Design review of the part built by this model. Coordinates are the model's own, in mm. Face numbers are marked on the shaded views. A direction names the side the tool comes from. Give positions to 0.01 mm unless a question says otherwise; leave off trailing zeros. Order: outer loops, then holes, each group sorted by start corner. A loop starts at its lowest first (then second) coordinate and runs counter-clockwise, first axis right, second up. Notation, with made-up numbers: (46.25, -20.75) -> (100.25, -20.75) arc R34 cw to (100.25, 13.25) -> close; hole circle Ø10 at (55.25, 16.25). An arc over 180 degrees is marked (long way). Use a Markdown table: item, result. Add a question column.
```python
from build123d import *

# Parameters (mm, degrees)
SKETCH1_W                = 177.8
SKETCH1_H                = 127
BOSS_EXTRUDE1_DEPTH      = 3.175
CONVERT_SOLID2_START     = -88.9
CONVERT_SOLID2_OUTLINE_W = 1.5875
CONVERT_SOLID2_OUTLINE_H = 127
CONVERT_SOLID2_DEPTH     = 177.8
EDGE_FLANGE1_DEPTH       = 177.8
EDGE_FLANGE2_DEPTH       = 177.8
SKETCH17_R               = 2.54
CUT_EXTRUDE1_DEPTH       = 5.08
FILLET1_R                = 12.7
SKETCH18_R               = 3.175
CUT_EXTRUDE2_DEPTH       = 5.08
SKETCH19_R               = 12.7
CUT_EXTRUDE3_DEPTH       = 12.7
SKETCH26_R               = 9.525
CUT_EXTRUDE9_DEPTH       = 5.08
SKETCH27_R               = 2.54
CUT_EXTRUDE10_DEPTH      = 5.08
SKETCH28_R               = 2.54
CUT_EXTRUDE11_DEPTH      = 5.08


# Read off the part's stored shape, not the designer's step: Convert-Solid2
# Sheet-metal steps are written as plain solids
with BuildPart() as part:
    # Sketch1 → Boss-Extrude1 (new body)
    with BuildSketch(Plane(origin=(0, 0, 0), x_dir=(1, 0, 0), z_dir=(0, 1, 0))):
        Rectangle(SKETCH1_W, SKETCH1_H)
    extrude(amount=BOSS_EXTRUDE1_DEPTH)

    # Convert-Solid2 outline → Convert-Solid2 (add)
    with BuildSketch(Plane.YZ.offset(CONVERT_SOLID2_START)):
        with Locations((-0.79375, 0)):
            Rectangle(CONVERT_SOLID2_OUTLINE_W, CONVERT_SOLID2_OUTLINE_H)
    extrude(amount=CONVERT_SOLID2_DEPTH)

    # Edge-Flange1 section (across the edge) → Edge-Flange1 (add)
    with BuildSketch(Plane(origin=(88.9, 3.175, -68.2625), x_dir=(0, 0, 1), z_dir=(-1, 0, 0))):
        with BuildLine():
            Line((-4.7625, 4.7625), (-4.7625, 33.3375))
            Line((-4.7625, 33.3375), (0, 33.3375))
            Line((0, 33.3375), (0, 4.7625))
            ThreePointArc((0, 4.7625), (1.394903955, 1.394903955), (4.7625, 0))
            Line((4.7625, 0), (4.7625, -4.7625))
            ThreePointArc((4.7625, -4.7625), (-1.972692091, -1.972692091), (-4.7625, 4.7625))
        make_face()
    extrude(amount=EDGE_FLANGE1_DEPTH)

    # Edge-Flange2 section (across the edge) → Edge-Flange2 (add)
    with BuildSketch(Plane(origin=(-88.9, 3.175, 68.2625), x_dir=(0, 0, -1), z_dir=(1, 0, 0))):
        with BuildLine():
            Line((-4.7625, 4.7625), (-4.7625, 33.3375))
            Line((-4.7625, 33.3375), (0, 33.3375))
            Line((0, 33.3375), (0, 4.7625))
            ThreePointArc((0, 4.7625), (1.394903955, 1.394903955), (4.7625, 0))
            Line((4.7625, 0), (4.7625, -4.7625))
            ThreePointArc((4.7625, -4.7625), (-1.972692091, -1.972692091), (-4.7625, 4.7625))
        make_face()
    extrude(amount=EDGE_FLANGE2_DEPTH)

    # Sketch17 → Cut-Extrude1 (cut)
    with BuildSketch(Plane(origin=(0, 0, -73.025), x_dir=(-1, 0, 0), z_dir=(0, 0, -1))):
        with Locations(Location((-76.2, 23.8125, 0), (0, 0, 90))):
            Circle(SKETCH17_R)
        with Locations(Location((-54.428571429, 23.8125, 0), (0, 0, 90))):
            Circle(SKETCH17_R)
        with Locations(Location((-32.657142857, 23.8125, 0), (0, 0, 90))):
            Circle(SKETCH17_R)
        with Locations(Location((-10.885714286, 23.8125, 0), (0, 0, 90))):
            Circle(SKETCH17_R)
        with Locations(Location((10.885714286, 23.8125, 0), (0, 0, 90))):
            Circle(SKETCH17_R)
        with Locations(Location((32.657142857, 23.8125, 0), (0, 0, 90))):
            Circle(SKETCH17_R)
        with Locations(Location((54.428571429, 23.8125, 0), (0, 0, 90))):
            Circle(SKETCH17_R)
        with Locations(Location((76.2, 23.8125, 0), (0, 0, 90))):
            Circle(SKETCH17_R)
    extrude(amount=-CUT_EXTRUDE1_DEPTH, mode=Mode.SUBTRACT)

    # Fillet1
    fillet1_edges = [part.edges().sort_by_distance(p)[0] for p in [
        (88.9, 36.5125, -70.64375),
        (-88.9, 36.5125, -70.64375),
        (-88.9, 36.5125, 70.64375),
        (88.9, 36.5125, 70.64375),
    ]]
    fillet(fillet1_edges, radius=FILLET1_R)

    # Sketch18 → Cut-Extrude2 (cut)
    with BuildSketch(Plane(origin=(0, 0, 68.2625), x_dir=(-1, 0, 0), z_dir=(0, 0, -1))):
        with Locations((69.85, 23.8125)):
            Circle(SKETCH18_R)
        with Locations((-69.85, 23.8125)):
            Circle(SKETCH18_R)
    extrude(amount=-CUT_EXTRUDE2_DEPTH, mode=Mode.SUBTRACT)

    # Sketch19 → Cut-Extrude3 (cut)
    with BuildSketch(Plane(origin=(0, -1.5875, 0), x_dir=(-1, 0, 0), z_dir=(0, -1, 0))):
        with Locations(Location((0, -12.7, 0), (0, 0, 90))):
            Circle(SKETCH19_R)
    extrude(amount=-CUT_EXTRUDE3_DEPTH, mode=Mode.SUBTRACT)

    # Sketch26 → Cut-Extrude9 (cut)
    with BuildSketch(Plane(origin=(0, -1.5875, 0), x_dir=(-1, 0, 0), z_dir=(0, -1, 0))):
        with Locations(Location((49.203281395, 25.4, 0), (0, 0, 90))):
            Circle(SKETCH26_R)
    extrude(amount=-CUT_EXTRUDE9_DEPTH, mode=Mode.SUBTRACT)

    # Sketch27 → Cut-Extrude10 (cut)
    with BuildSketch(Plane.XZ.offset(1.5875)):
        with Locations(Location((-23.803281395, -25.4, 0), (0, 0, 270))):
            Circle(SKETCH27_R)
    extrude(amount=-CUT_EXTRUDE10_DEPTH, mode=Mode.SUBTRACT)

    # Sketch28 → Cut-Extrude11 (cut)
    with BuildSketch(Plane(origin=(0, -1.5875, 0), x_dir=(-1, 0, 0), z_dir=(0, -1, 0))):
        with Locations(Location((74.603281395, 25.4, 0), (0, 0, 90))):
            Circle(SKETCH28_R)
    extrude(amount=-CUT_EXTRUDE11_DEPTH, mode=Mode.SUBTRACT)


solid = part.part
```
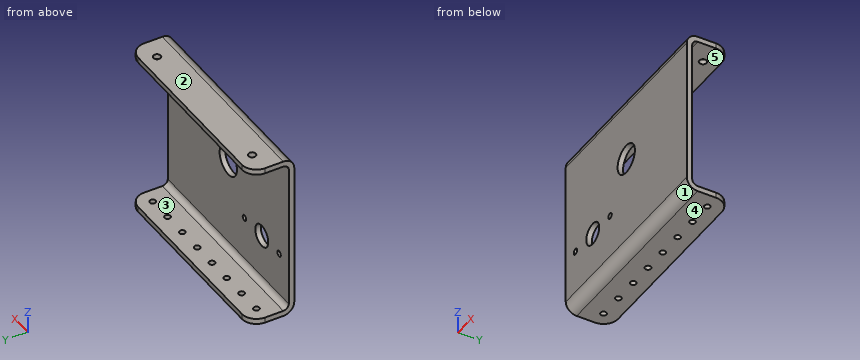
1) The part is to be moulded in two halves that separate along Z. For the marked faces 1, 2 and 3, say which applies: +Z half, -Z half, draft (parallel to the pull), parting line (faces both ways), or undercut.
2) For L1, parallel to X at y = 1, z = -25; L2, parallel to X at y = 0, z = 12; L3, parallel to Z at x = -34.5, y = 11.5 (1 decimal), list the stretches that pass through material, from the lowest coordinate up. Write a range as [from, to].
3) Add section A-A (z = 12.7). Give the boundary of the cut face in (x, y) (1 decimal).
4) Add section D-D (z = -25.4). Give the boundary of the cut face in (x, y) (1 decimal), then the cut area to 3 significant figures.
5) Machinability: for the marked faces 4 and 5, which of the approach directions +Z, -Z, +X, -X, +Y, -Y give a long, thin tool a straight path to every point of the face, cutting with its end or side? Answer none if there is none.
6) Insertion check: pin 1 (5 mm diameter, centred on x = -5.5, z = -8.5, fed in from +Y) (3 decimals); pin 2 (3 mm diameter, centred on x = -32.66, y = 23.81, fed in from -Z). Each pin has a flat end and moves straight along its axis. Give the tip position at first contact, or say it passes through.
Worked answers:
| question | item | result |
|---|---|---|
| 1 | face 1 | -Z half |
| 1 | face 2 | +Z half |
| 1 | face 3 | undercut |
| 2 | L1 | [-88.9, -77.11], [-72.09, -58.72], [-39.69, -26.31], [-21.29, 88.9] |
| 2 | L2 | [-88.9, -12.68], [12.68, 88.9] |
| 2 | L3 | [-73, -68.3], [68.3, 73] |
| 3 | outline | (-88.9, -1.6) -> (-12.7, -1.6) -> (-12.7, 3.2) -> (-88.9, 3.2) -> close; (12.7, -1.6) -> (88.9, -1.6) -> (88.9, 3.2) -> (12.7, 3.2) -> close |
| 4 | outline | (-88.9, -1.6) -> (-77.1, -1.6) -> (-77.1, 3.2) -> (-88.9, 3.2) -> close; (-72.1, -1.6) -> (-58.7, -1.6) -> (-58.7, 3.2) -> (-72.1, 3.2) -> close; (-39.7, -1.6) -> (-26.3, -1.6) -> (-26.3, 3.2) -> (-39.7, 3.2) -> close; (-21.3, -1.6) -> (88.9, -1.6) -> (88.9, 3.2) -> (-21.3, 3.2) -> close |
| 4 | area | 708 mm^2 |
| 5 | face 4 | -Z, +X, -X, +Y, -Y |
| 5 | face 5 | +X, -X, +Y |
| 6 | pin 1 | y = 3.175 |
| 6 | pin 2 | z = 68.26 |
